from build123d import *

# Parameters (mm, degrees)
SM_BASE_FLANGE_1_DEPTH = 100
SKETCH_4_R             = 4.05
CUT_EXTRUDE_1_DEPTH    = 116.905133622
SKETCH_5_W             = 10
SKETCH_5_H             = 9
SKETCH_5_W_2           = 14
CUT_EXTRUDE_2_DEPTH    = 116.905133622
FILLET_1_R             = 6
SKETCH_7_W             = 8.2
SKETCH_7_H             = 8.2
CUT_EXTRUDE_4_DEPTH    = 4
CUT_EXTRUDE_5_DEPTH    = 4


# Sheet-metal steps are written as plain solids
with BuildPart() as part:
    # Sketch 1 → Базовая кромка1 (new body)
    with BuildSketch(Plane(origin=(0, 0, 0), x_dir=(0, 0, -1), z_dir=(1, 0, 0))):
        with BuildLine():
            Line((-25, -53), (-9, -53))
            ThreePointArc((-9, -53), (-2.636038969, -50.363961031), (0, -44))
            Line((0, -44), (0, -9))
            ThreePointArc((0, -9), (-2.636038969, -2.636038969), (-9, 0))
            Line((-9, 0), (-25, 0))
            Line((-25, 0), (-25, -4))
            Line((-25, -4), (-9, -4))
            ThreePointArc((-9, -4), (-5.464466094, -5.464466094), (-4, -9))
            Line((-4, -9), (-4, -44))
            ThreePointArc((-4, -44), (-5.464466094, -47.535533906), (-9, -49))
            Line((-9, -49), (-25, -49))
            Line((-25, -49), (-25, -53))
        make_face()
    extrude(amount=SM_BASE_FLANGE_1_DEPTH)

    # Эскиз4 → Вырез-Вытянуть1 (cut, through all)
    with BuildSketch(Plane(origin=(0, 0, 0), x_dir=(1, 0, 0), z_dir=(0, 1, 0))):
        with Locations(Location((12, -17, 0), (0, 0, 270))):
            Circle(SKETCH_4_R)
        with Locations(Location((92, -17, 0), (0, 0, 270))):
            Circle(SKETCH_4_R)
    extrude(amount=-CUT_EXTRUDE_1_DEPTH, mode=Mode.SUBTRACT)

    # Эскиз5 → Вырез-Вытянуть2 (cut, through all)
    with BuildSketch(Plane(origin=(0, 0, 0), x_dir=(1, 0, 0), z_dir=(0, 1, 0))):
        with Locations((5, -4.5)):
            Rectangle(SKETCH_5_W, SKETCH_5_H)
        with Locations((93, -4.5)):
            Rectangle(SKETCH_5_W_2, SKETCH_5_H)
    extrude(amount=-CUT_EXTRUDE_2_DEPTH, mode=Mode.SUBTRACT)

    # Скругление1
    fillet_1_edges = [part.edges().sort_by_distance(p)[0] for p in [
        (0, -51, 25),
        (0, -2, 25),
        (100, -51, 25),
        (0, -2, 9),
        (100, -2, 9),
        (0, -51, 9),
        (100, -51, 9),
        (100, -2, 25),
    ]]
    fillet(fillet_1_edges, radius=FILLET_1_R)

    # Эскиз7 → Вырез-Вытянуть4 (cut)
    with BuildSketch(Plane.XZ.offset(53)):
        with Locations((12, 17)):
            Rectangle(SKETCH_7_W, SKETCH_7_H)
    extrude(amount=-CUT_EXTRUDE_4_DEPTH, mode=Mode.SUBTRACT)

    # Эскиз8 → Вырез-Вытянуть5 (cut)
    with BuildSketch(Plane(origin=(0, 0, 0), x_dir=(-1, 0, 0), z_dir=(0, 0, -1))):
        with BuildLine():
            Line((-69.5, -17.5), (-62.5, -17.5))
            ThreePointArc((-62.5, -17.5), (-61, -19), (-62.5, -20.5))
            Line((-62.5, -20.5), (-69.5, -20.5))
            ThreePointArc((-69.5, -20.5), (-71, -19), (-69.5, -17.5))
        make_face()
        with BuildLine():
            Line((-26.5, -17.5), (-33.5, -17.5))
            ThreePointArc((-33.5, -17.5), (-35, -19), (-33.5, -20.5))
            Line((-33.5, -20.5), (-26.5, -20.5))
            ThreePointArc((-26.5, -20.5), (-25, -19), (-26.5, -17.5))
        make_face()
        with BuildLine():
            Line((-26.5, -35.5), (-33.5, -35.5))
            ThreePointArc((-33.5, -35.5), (-35, -34), (-33.5, -32.5))
            Line((-33.5, -32.5), (-26.5, -32.5))
            ThreePointArc((-26.5, -32.5), (-25, -34), (-26.5, -35.5))
        make_face()
        with BuildLine():
            Line((-69.5, -35.5), (-62.5, -35.5))
            ThreePointArc((-62.5, -35.5), (-61, -34), (-62.5, -32.5))
            Line((-62.5, -32.5), (-69.5, -32.5))
            ThreePointArc((-69.5, -32.5), (-71, -34), (-69.5, -35.5))
        make_face()
    extrude(amount=-CUT_EXTRUDE_5_DEPTH, mode=Mode.SUBTRACT)


solid = part.part
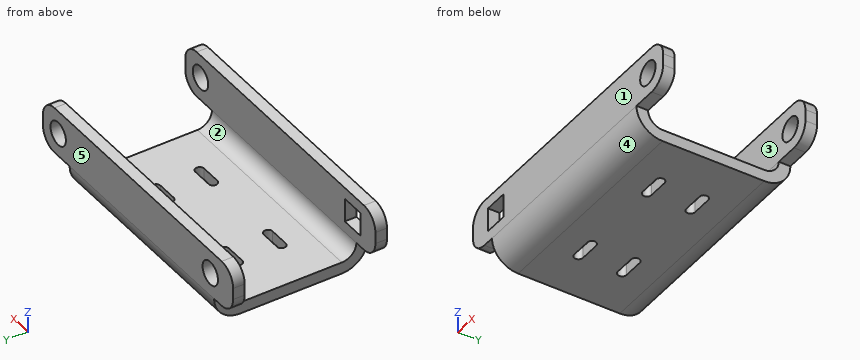
Here's how the part is built. I have some questions about the finished solid (model axes, mm). Face numbers are marked on the shaded views. A direction names the side the tool comes from. Round coordinates to 2 decimals unless told otherwise and drop trailing zeros. Order: outer loops, then holes, each group sorted by start corner. A loop starts at its lowest first (then second) coordinate and runs counter-clockwise, first axis right, second up. Notation, with made-up numbers: (-9, 31) -> (-2, 31) arc R16 cw to (-2, 55) -> close; hole circle Ø11 at (24.5, 36.5). An arc over 180 degrees is marked (long way). Return JSON: item names as keys, results as strings.
Q1. If we section it at A-A on x = 92: List the corners of the cut face in (y, z) for me, plus the area to 3 significant figures.
Filled sheet:
{"outline": "(-53, 9) -> (-49, 9) -> (-49, 12.95) -> (-53, 12.95) -> close; (-53, 21.05) -> (-49, 21.05) -> (-49, 25) -> (-53, 25) -> close; (-4, 9) -> (0, 9) -> (0, 12.95) -> (-4, 12.95) -> close; (-4, 21.05) -> (0, 21.05) -> (0, 25) -> (-4, 25) -> close", "area": "63.2 mm^2"}
Q2. For pin 1 Ø3 at (x, z) = (31, 3) entering from -Y; pin 2 Ø9.5 at (x, z) = (92, 17) entering from +Y; pin 3 Ø3 at (x, z) = (31.5, 2.5) entering from -Y; pin 4 Ø6 at (x, y) = (52, -20.5) entering from +Z, each with a flat end and sliding along its axis, tell me the tip position at first contact or that it passes through.
Filled sheet:
{"pin 1": "stops at y = -51.79", "pin 2": "stops at y = 0", "pin 3": "stops at y = -51.48", "pin 4": "stops at z = 4"}
Q3. I need wall thicknesses on line 1 along X through (y, z) = (-2.9, 17); line 2 along X through (y, z) = (-50.1, 17); line 3 along Y through (x, z) = (45, 14.5). Which ranges of each line are inside material? Lowest first, please. Write a range as from..to.
Filled sheet:
{"line 1": "x = 0..7.95, 16.05..87.95, 96.05..100", "line 2": "x = 0..7.9, 16.1..87.95, 96.05..100", "line 3": "y = -53..-49, -4..0"}
Q4. If we section it at C-C on y = -34: List the corners of the cut face in (x, z) for me.
Filled sheet:
{"outline": "(10, 0) -> (25, 0) -> (25, 4) -> (10, 4) -> close; (35, 0) -> (61, 0) -> (61, 4) -> (35, 4) -> close; (71, 0) -> (86, 0) -> (86, 4) -> (71, 4) -> close"}
Q5. If we mould it in two halves opening along Y, with no side actions, what happens to the marked faces 3, 4 and 5? For each: released by +Y, released by -Y, zero draft, split by the parting line, or undercut.
Filled sheet:
{"face 3": "undercut", "face 4": "released by -Y", "face 5": "released by +Y"}
Q6. Which directions (+Z, -Z, +X, -X, +Y, -Y) give clear straight access to the entire face, cutting with the end or side of a thin tool? Please do the marked faces 1 and 2.
Filled sheet:
{"face 1": "+Z, -Z, +X, -X, -Y", "face 2": "+Z, +X, -X"}
Q7. If we section it at B-B on z = 17: List the corners of the cut face in (x, y) for me, plus the area to 3 significant figures.
Filled sheet:
{"outline": "(0, -53) -> (7.9, -53) -> (7.9, -49) -> (0, -49) -> close; (0, -4) -> (7.95, -4) -> (7.95, 0) -> (0, 0) -> close; (16.05, -4) -> (87.95, -4) -> (87.95, 0) -> (16.05, 0) -> close; (16.1, -53) -> (87.95, -53) -> (87.95, -49) -> (16.1, -49) -> close; (96.05, -53) -> (100, -53) -> (100, -49) -> (96.05, -49) -> close; (96.05, -4) -> (100, -4) -> (100, 0) -> (96.05, 0) -> close", "area": "670 mm^2"}
Q8. If we section it at D-D on z = 23: List the corners of the cut face in (x, y) for me.
Filled sheet:
{"outline": "(1.53, -53) -> (98.47, -53) -> (98.47, -49) -> (1.53, -49) -> close; (1.53, -4) -> (98.47, -4) -> (98.47, 0) -> (1.53, 0) -> close"}
